```python
from build123d import *

# Parameters (mm, degrees)
SKETCH1_R           = 23.25
SKETCH1_R_2         = 21.25
BOSS_EXTRUDE1_DEPTH = 30
SKETCH1_4_R         = 33
SKETCH1_4_R_2       = 23.25
BOSS_EXTRUDE2_DEPTH = 3
SKETCH2_R           = 1.7
CUT_EXTRUDE1_DEPTH  = 54.916602267


with BuildPart() as part:
    # Sketch1 → Boss-Extrude1 (new body)
    with BuildSketch(Plane(origin=(0, 0, 0), x_dir=(1, 0, 0), z_dir=(0, 1, 0))):
        with Locations(Location((0, 0, 0), (0, 0, 270))):
            Circle(SKETCH1_R)
        with Locations(Location((0, 0, 0), (0, 0, 270))):
            Circle(SKETCH1_R_2, mode=Mode.SUBTRACT)
    extrude(amount=BOSS_EXTRUDE1_DEPTH)

    # Sketch1_4 → Boss-Extrude2 (add)
    with BuildSketch(Plane(origin=(0, 0, 0), x_dir=(1, 0, 0), z_dir=(0, 1, 0))):
        with Locations(Location((0, 0, 0), (0, 0, 270))):
            Circle(SKETCH1_4_R)
        with Locations(Location((0, 0, 0), (0, 0, 270))):
            Circle(SKETCH1_4_R_2, mode=Mode.SUBTRACT)
    extrude(amount=BOSS_EXTRUDE2_DEPTH)

    # Sketch2 → Cut-Extrude1 (cut, through all)
    with BuildSketch(Plane(origin=(0, 3, 0), x_dir=(1, 0, 0), z_dir=(0, 1, 0))):
        with Locations(Location((27, 0, 0), (0, 0, 270))):
            Circle(SKETCH2_R)
        with Locations(Location((-13.5, -23.382685902, 0), (0, 0, 270))):
            Circle(SKETCH2_R)
        with Locations(Location((-13.5, 23.382685902, 0), (0, 0, 270))):
            Circle(SKETCH2_R)
    extrude(amount=-CUT_EXTRUDE1_DEPTH, mode=Mode.SUBTRACT)


solid = part.part
```
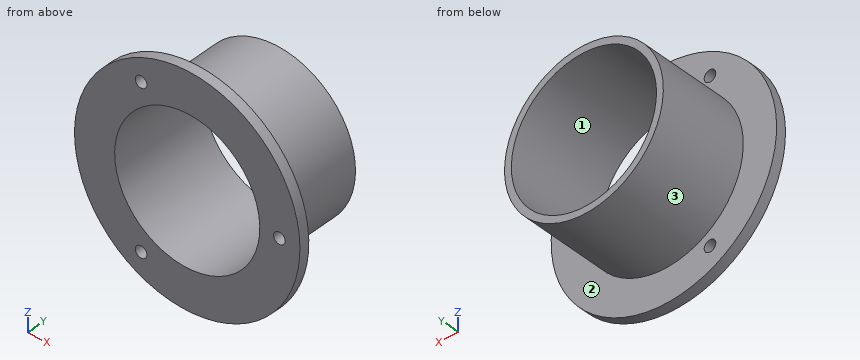
Read the model definition and answer for the solid it produces. Units are mm, in the model's axes. Face numbers are marked on the shaded views. Round coordinates to 2 decimals unless told otherwise and drop trailing zeros. Write each loop counter-clockwise with the first axis right and the second up, starting at its lowest first coordinate (ties: lowest second). Pieces come first, ordered by that corner, then holes. Notation, with made-up numbers: (-18, 59) -> (13, 59) arc R23 cw to (13, 98) -> close; hole circle Ø11 at (-12.75, 21). An arc over 180 degrees is marked (long way). Answer in a Markdown table with one row per item. Add a question column.
1) Find section C-C, the plane z = 11.5. Determine the outline of the cut face in (x, y), and give its area (3 significant figures).
2) Given P1, Ø5.5, axis at x = -13.5, z = -23.38, coming from the +Y side; P2, Ø3, axis at x = 27, z = 0, coming from the +Y side; P3, Ø6, axis at x = -0.5, y = 7.5, coming from the -Z side; P4, Ø12, axis at y = 4, z = -22.5, coming from the +X side, each flat-ended and moving along its own axis, determine where each tip first touches the part or whether it passes through.
3) Consider line 1 (X direction, y = 0.9, z = 0); line 2 (Y direction, x = -1.5, z = -27); line 3 (Z direction, x = 2, y = 11.5). Determine where each line is inside the solid, lowest interval first.
4) Find section A-A, the plane z = 0. Determine the outline of the cut face in (x, y).
5) Determine the mould class of the marked faces 1, 2 and 3 for opening direction X: pulls with the +X half, pulls with the -X half, needs draft (parallel to the pull), parting line crosses it, or undercut.
6) Find section D-D, the plane y = 25.25. Determine the outline of the cut face in (x, z), and give its area (3 significant figures).
7) Find section B-B, the plane x = 0. Determine the outline of the cut face in (y, z), and give its area (4 significant figures).
Findings below:
| question | item | result |
|---|---|---|
| 1 | outline | (-30.93, 0) -> (-17.87, 0) -> (-17.87, 30) -> (-20.21, 30) -> (-20.21, 3) -> (-30.93, 3) -> close; (17.87, 0) -> (30.93, 0) -> (30.93, 3) -> (20.21, 3) -> (20.21, 30) -> (17.87, 30) -> close |
| 1 | area | 205 mm² |
| 2 | P1 | y = 3 |
| 2 | P2 | through |
| 2 | P3 | z = -23.25 |
| 2 | P4 | x = 28.53 |
| 3 | line 1 | -33 to -21.25, 21.25 to 25.3, 28.7 to 33 |
| 3 | line 2 | 0 to 3 |
| 3 | line 3 | -23.16 to -21.16, 21.16 to 23.16 |
| 4 | outline | (-33, 0) -> (-21.25, 0) -> (-21.25, 30) -> (-23.25, 30) -> (-23.25, 3) -> (-33, 3) -> close; (21.25, 0) -> (25.3, 0) -> (25.3, 3) -> (23.25, 3) -> (23.25, 30) -> (21.25, 30) -> close; (28.7, 0) -> (33, 0) -> (33, 3) -> (28.7, 3) -> close |
| 5 | face 1 | undercut |
| 5 | face 2 | needs draft |
| 5 | face 3 | parting line crosses it |
| 6 | outline | circle Ø46.5 at (0, 0); hole circle Ø42.5 at (0, 0) |
| 6 | area | 280 mm² |
| 7 | outline | (0, -33) -> (3, -33) -> (3, -23.25) -> (30, -23.25) -> (30, -21.25) -> (0, -21.25) -> close; (0, 21.25) -> (30, 21.25) -> (30, 23.25) -> (3, 23.25) -> (3, 33) -> (0, 33) -> close |
| 7 | area | 178.5 mm² |
